Part print with two shaded views. Sizes in mm from the minimum x, y, z corner. A direction names the side the tool comes from. Give positions to 0.01 mm unless a question says otherwise; leave off trailing zeros. Write each loop counter-clockwise with the first axis right and the second up, starting at its lowest first coordinate (ties: lowest second). Pieces come first, ordered by that corner, then holes.
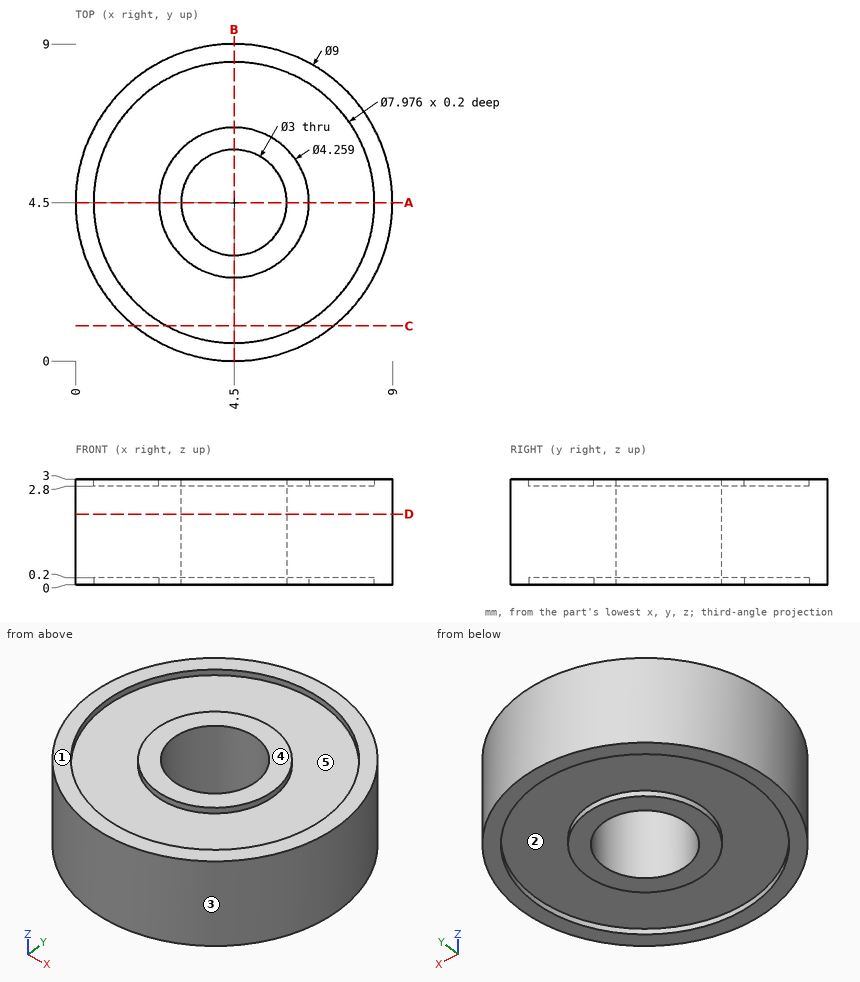
1) 3-axis set-ups, long thin cutter, end or side, ignore diameter. For the marked faces 4 and 5: which of +Z, -Z, +X, -X, +Y, -Y reach the whole face in a straight line?
Check result:
face 4: +Z, +X, -X, +Y, -Y
face 5: +Z
2) Mould opens along X. For the marked faces 1, 2 and 3 say: +X half, -X half, draft (parallel to the pull), parting line (faces both ways), or undercut.
Check result:
face 1: draft
face 2: undercut
face 3: parting line
3) Drill centre lines: L1, parallel to Y at x = 4.5, z = 2.9; L2, parallel to Y at x = 4.5, z = 2.1; L3, parallel to Z at x = 7.5, y = 6. Where is each one in solid material? Low to high.
Check result:
L1: y = 0 to 0.51, 2.37 to 3, 6 to 6.63, 8.49 to 9
L2: y = 0 to 3, 6 to 9
L3: z = 0.2 to 2.8
4) Saw through at D-D (z = 2). Write the cut outline in (x, y).
Check result:
outline: circle Ø9 at (4.5, 4.5); hole circle Ø3 at (4.5, 4.5)
5) Flat gauge pins, fed straight in: P1, Ø1, axis at x = 6, z = 1.5, coming from the +Y side; P2, Ø1, axis at y = 7, z = 2.5, coming from the -X side. Where does each tip first touch, or does it go through?
Check result:
P1: stops at y = 8.89
P2: stops at x = 0.47
6) Saw through at C-C (y = 1). Write the cut outline in (x, z).
Check result:
outline: (1.67, 0) - (2.59, 0) - (2.59, 0.2) - (6.41, 0.2) - (6.41, 0) - (7.33, 0) - (7.33, 3) - (6.41, 3) - (6.41, 2.8) - (2.59, 2.8) - (2.59, 3) - (1.67, 3) - close
7) Saw through at A-A (y = 4.5). Write the cut outline in (x, z).
Check result:
outline: (0, 0) - (0.51, 0) - (0.51, 0.2) - (2.37, 0.2) - (2.37, 0) - (3, 0) - (3, 3) - (2.37, 3) - (2.37, 2.8) - (0.51, 2.8) - (0.51, 3) - (0, 3) - close; (6, 0) - (6.63, 0) - (6.63, 0.2) - (8.49, 0.2) - (8.49, 0) - (9, 0) - (9, 3) - (8.49, 3) - (8.49, 2.8) - (6.63, 2.8) - (6.63, 3) - (6, 3) - close
